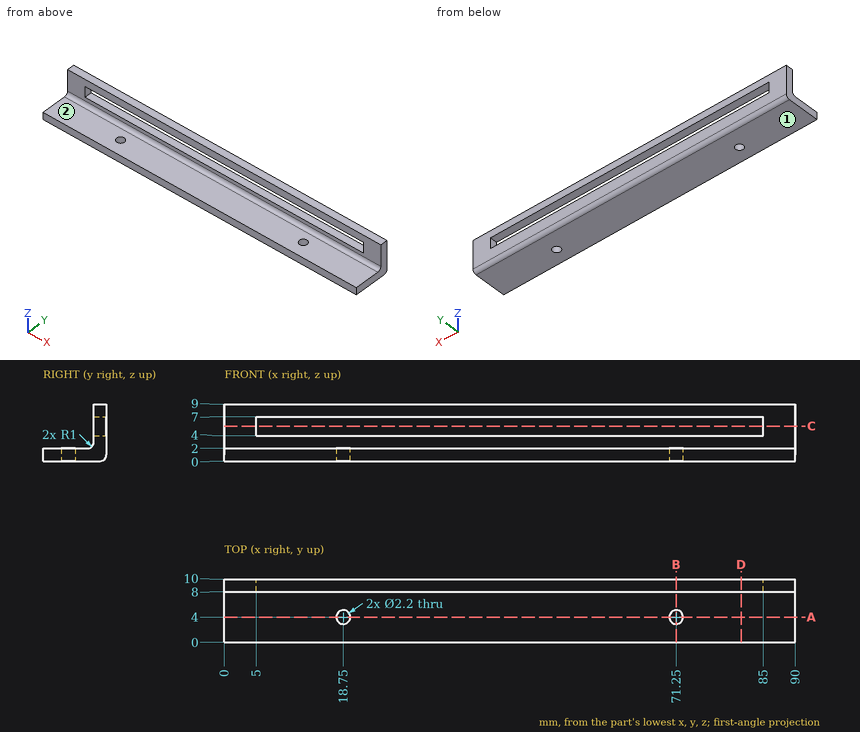
Job drawing, mm, ordinate dimensions from the low corner. One solid piece. A direction names the side the tool comes from. Round coordinates to 2 decimals unless told otherwise and drop trailing zeros. Loops run counter-clockwise (first coordinate to the right, second up) from the corner with the lowest first, then second, coordinate; pieces in that order, holes last. Notation, with made-up numbers: (-26.5, 15) -> (-7.5, 15) arc R18 cw to (-7.5, 44) -> close; hole circle Ø9 at (12, 60.25). An arc over 180 degrees is marked (long way). Use a Markdown table: item, result.
1) Cut at B-B, the plane x = 71.25. List the corners of the cut face in (y, z), and give its area (3 significant figures).
The answers:
| item | result |
|---|---|
| outline | (0, 0) -> (2.9, 0) -> (2.9, 2) -> (0, 2) -> close; (5.1, 0) -> (9, 0) arc R1 ccw to (10, 1) -> (10, 4) -> (8, 4) -> (8, 3) arc R1 cw to (7, 2) -> (5.1, 2) -> close; (8, 7) -> (10, 7) -> (10, 9) -> (8, 9) -> close |
| area | 23.6 mm2 |
2) Tool access for the marked faces 1 and 2: list every direction of +Z, -Z, +X, -X, +Y, -Y with a clear straight run to the whole face (end or side of a thin tool).
The answers:
| item | result |
|---|---|
| face 1 | -Z, +X, -X, +Y, -Y |
| face 2 | +Z, +X, -X, -Y |
3) Probe line 1 (Y direction, x = 71.25, z = 1.4); line 2 (Z direction, x = 55.5, y = 9); line 3 (Y direction, x = 10, z = 3.25). List the from-to ranges inside material, lowest first. Write a range as [from, to].
The answers:
| item | result |
|---|---|
| line 1 | y = [0, 2.9], [5.1, 10] |
| line 2 | z = [0, 4], [7, 9] |
| line 3 | y = [8, 10] |
4) Cut at D-D, the plane x = 81.5. List the corners of the cut face in (y, z).
The answers:
| item | result |
|---|---|
| outline | (0, 0) -> (9, 0) arc R1 ccw to (10, 1) -> (10, 4) -> (8, 4) -> (8, 3) arc R1 cw to (7, 2) -> (0, 2) -> close; (8, 7) -> (10, 7) -> (10, 9) -> (8, 9) -> close |
5) Cut at C-C, the plane z = 5.5. List the corners of the cut face in (x, y), and give its area (3 significant figures).
The answers:
| item | result |
|---|---|
| outline | (0, 8) -> (5, 8) -> (5, 10) -> (0, 10) -> close; (85, 8) -> (90, 8) -> (90, 10) -> (85, 10) -> close |
| area | 20.0 mm2 |
6) Drop flat-ended pins along their axis: pin 1 Ø1.5 at (x, z) = (18, 3.5) entering from -Y; pin 2 Ø3.5 at (x, y) = (18.75, 4) entering from +Z; pin 3 Ø1.8 at (x, y) = (71.25, 4) entering from +Z. Give the stop position or say it passes through.
The answers:
| item | result |
|---|---|
| pin 1 | stops at y = 7.97 |
| pin 2 | stops at z = 2 |
| pin 3 | passes through |
7) Cut at A-A, the plane y = 4. List the corners of the cut face in (x, z).
The answers:
| item | result |
|---|---|
| outline | (0, 0) -> (17.65, 0) -> (17.65, 2) -> (0, 2) -> close; (19.85, 0) -> (70.15, 0) -> (70.15, 2) -> (19.85, 2) -> close; (72.35, 0) -> (90, 0) -> (90, 2) -> (72.35, 2) -> close |
